Autodesk Inventor part; units mm, degrees
ref_plane "YZ Plane" through (0, 0, 0) normal (1, 0, 0) x (0, 1, 0)
ref_plane "XZ Plane" through (0, 0, 0) normal (0, 1, 0) x (-1, 0, 0)
ref_plane "XY Plane" through (0, 0, 0) normal (0, 0, 1) x (1, 0, 0)
sketch "Sketch1" plane through (0, 0, 0) normal (0, 0, 1) x (1, 0, 0)
  circle A0 centre (0, 0) radius 20.6
  circle A1 centre (0, 0) radius 22.4
  dimension "d0" = 41.2
  dimension "d1" = 1.8
extrude "Extrusion1" add sketch "Sketch1" along normal blind 2 contours A0 | A1
extrude "Extrusion2" add sketch "Sketch1" along normal blind 8
sketch "Sketch2" plane through (0, 0, 2) normal (0, 0, 1) x (1, 0, 0)
  line L0 (-1.5, 12.5) -> (1.5, 12.5)
  line L1 (1.5, 12.5) -> (1.5, -12.5)
  line L2 (1.5, -12.5) -> (-1.5, -12.5)
  line L3 (-1.5, -12.5) -> (-1.5, 12.5)
  point P0 (0, 0)
  point P1 (0, 12.5)
  point P2 (1.5, 0)
  dimension "d6" = 3
  dimension "d7" = 25
extrude "Extrusion3" cut sketch "Sketch2" against normal through all
sketch "Sketch3" plane through (0, 0, 2) normal (0, 0, 1) x (1, 0, 0)
  line L0 (1.5, 12.5) -> (1.5, -12.5)
  line L1 (1.5, 12.5) -> (10.8, 12.5)
  line L2 (10.8, 12.5) -> (10.8, -12.5)
  line L3 (10.8, -12.5) -> (1.5, -12.5)
  line L4 (1.5, -12.5) -> (1.5, 12.5)
  point P0 (0, 0)
  dimension "d10" = 9.3
extrude "Extrusion4" cut sketch "Sketch3" against normal blind 0.4
mirror "Mirror1" about plane through (0, 0, 0) normal (1, 0, 0) of "Extrusion4"
chamfer "Chamfer1" distance 1 angle 45 2 edges at (1.5, 0, 0) (-1.5, 0, 0)
fillet "Fillet1" radius 0.4 4 edges at (-1.5, -12.5, 1.3) (1.5, -12.5, 1.3) (-1.5, 12.5, 1.3) (1.5, 12.5, 1.3)
fillet "Fillet2" radius 1 4 edges at (-10.8, 12.5, 1.8) (10.8, 12.5, 1.8) (10.8, -12.5, 1.8) (-10.8, -12.5, 1.8)
chamfer "Chamfer2" distance 0.4 angle 45 6 edges at (-22.4, 0, 8) (-20.6, 0, 8) (-20.6, 0, 2) (-22.4, 0, 0) (0, 12.5, 0) (0, -12.5, 0)
sketch "Sketch4" plane through (0, 0, 0) normal (0, 0, -1) x (-1, 0, 0)
  line L0 (15, 0) -> (-15, 0) construction
  point P0 (0, 0)
  point P1 (0, 0)
  dimension "d21" = 30
hole "Hole1" at (-15, 0, 0) at (15, 0, 0) direction (0, 0, 1) diameter 2.9 end through all
chamfer "Chamfer3" distance 0.4 angle 45 4 edges at (15, -1.45, 0) (-15, -1.45, 0) (15, -1.45, 2) (-15, -1.45, 2)
properties part number "takumar-slit" material "ABS Plastic"
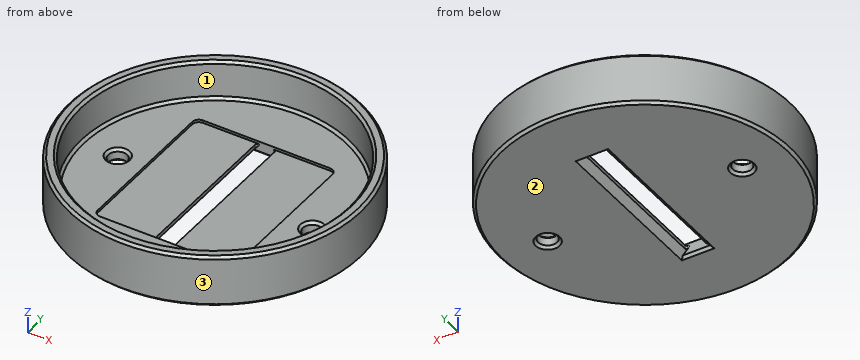
Read the model definition and answer for the solid it produces. Units are mm, in the model's axes. Face numbers are marked on the shaded views. Give positions to 0.01 mm unless a question says otherwise; leave off trailing zeros. Write each loop counter-clockwise with the first axis right and the second up, starting at its lowest first coordinate (ties: lowest second). Pieces come first, ordered by that corner, then holes. Notation, with made-up numbers: (-28, 33) - (16, 33) arc R18 cw to (16, 42) - close; hole circle Ø5 at (-29, 76). An arc over 180 degrees is marked (long way). Return JSON: item names as keys, results as strings.
Q1. Given P1, Ø0.5, axis at x = -3.5, z = 1.5, coming from the +Y side; P2, Ø1, axis at y = 8, z = 2, coming from the -X side; P3, Ø10.5, axis at x = 5.5, y = -2.5, coming from the +Z side, each flat-ended and moving along its own axis, determine where each tip first touches the part or whether it passes through.
Reply:
{"P1": "y = 22.16", "P2": "x = -21.11", "P3": "z = 1.6"}
Q2. A cutting plane is placed at A-A, the plane x = 0. Determine the outline of the cut face in (y, z), and give its area (3 significant figures).
Reply:
{"outline": "(-22.4, 0.4) - (-22, 0) - (-12.9, 0) - (-12.5, 0.4) - (-12.5, 2) - (-20.2, 2) - (-20.6, 2.4) - (-20.6, 7.6) - (-21, 8) - (-22, 8) - (-22.4, 7.6) - close; (12.5, 0.4) - (12.9, 0) - (22, 0) - (22.4, 0.4) - (22.4, 7.6) - (22, 8) - (21, 8) - (20.6, 7.6) - (20.6, 2.4) - (20.2, 2) - (12.5, 2) - close", "area": "60.7 mm²"}
Q3. Consider line 1 along Z through (x, y) = (9, 16); line 2 along Z through (x, y) = (10, 7); line 3 along X through (y, z) = (-5, 5.75). Determine where each line is inside the solid, lowest interval first. Write a range as [from, to].
Reply:
{"line 1": "[0, 2]", "line 2": "[0, 1.6]", "line 3": "[-21.83, -19.98], [19.98, 21.83]"}
Q4. A cutting plane is placed at B-B, the plane z = 5.5. Determine the outline of the cut face in (x, y).
Reply:
{"outline": "circle Ø44.8 at (0, 0); hole circle Ø41.2 at (0, 0)"}
Q5. A cutting plane is placed at C-C, the plane y = 0. Count the separate pieces of the cut face and the enclosed holes in it, and give its area (3 significant figures).
Reply:
{"separate pieces": "4", "enclosed holes": "0", "area": "84.2 mm²"}
Q6. For a pull along X with two mould halves and no side action, classify the marked faces 1, 2 and 3 as released by +X, released by -X, zero draft, split by the parting line, or undercut.
Reply:
{"face 1": "undercut", "face 2": "zero draft", "face 3": "split by the parting line"}
